```python
from build123d import *

# Parameters (mm, degrees)
SKETCH2_W           = 30
SKETCH2_H           = 30
BOSS_EXTRUDE1_DEPTH = 6.35
FILLET1_R           = 10
SKETCH3_R           = 6.5
BOSS_EXTRUDE2_DEPTH = 50
SKETCH4_R           = 0.5
BOSS_EXTRUDE3_DEPTH = 20
FILLET2_R           = 0.5
CHAMFER1_SIZE       = 6.5


with BuildPart() as part:
    # Sketch2 → Boss-Extrude1 (new body)
    with BuildSketch(Plane(origin=(0, 0, 0), x_dir=(1, 0, 0), z_dir=(0, 1, 0))):
        Rectangle(SKETCH2_W, SKETCH2_H)
    extrude(amount=BOSS_EXTRUDE1_DEPTH)

    # Fillet1
    fillet1_edges = [part.edges().sort_by_distance(p)[0] for p in [
        (-15, 3.175, 15),
        (-15, 3.175, -15),
        (15, 3.175, -15),
        (15, 3.175, 15),
    ]]
    fillet(fillet1_edges, radius=FILLET1_R)

    # Sketch3 → Boss-Extrude2 (add)
    with BuildSketch(Plane(origin=(0, 6.35, 0), x_dir=(1, 0, 0), z_dir=(0, 1, 0))):
        with Locations(Location((0, 0, 0), (0, 0, 270))):
            Circle(SKETCH3_R)
    extrude(amount=BOSS_EXTRUDE2_DEPTH)

    # Sketch4 → Boss-Extrude3 (add)
    with BuildSketch(Plane(origin=(0, 56.35, 0), x_dir=(1, 0, 0), z_dir=(0, 1, 0))):
        with Locations(Location((0, 0, 0), (0, 0, 270))):
            Circle(SKETCH4_R)
    extrude(amount=BOSS_EXTRUDE3_DEPTH)

    # Fillet2
    fillet2_edges = [part.edges().sort_by_distance(p)[0] for p in [
        (0, 76.35, -0.5),
    ]]
    fillet(fillet2_edges, radius=FILLET2_R)

    # Chamfer1
    # the kernel refuses this chamfer: 6.5 mm, written as the material it adds along each edge
    with BuildSketch(Plane(origin=(0, 56.35, 0), x_dir=(0, 0, 1), z_dir=(-1, 0, 0))) as chamfer1_piece_1_section:
        Polygon((0.5, CHAMFER1_SIZE), (0.5 + CHAMFER1_SIZE, 0), (0.5, 0), align=None)
    chamfer1_piece_1 = revolve(axis=Axis((0, 56.35, 0), (0, 1, 0)), mode=Mode.PRIVATE)
    chamfer1_piece_1 = chamfer1_piece_1 & Plane(origin=(0, 59.89101351, 0), x_dir=(0, 0, 1), z_dir=(0, -1, 0)) * Cylinder(6.5, 28, mode=Mode.PRIVATE)
    add(chamfer1_piece_1)


solid = part.part
```
Can you work these out from the model? Positions are in its coordinate system, mm. A direction names the side the tool comes from. Coordinates: 2 decimals unless noted, no trailing zeros. Order: outer loops, then holes, each group sorted by start corner. A loop starts at its lowest first (then second) coordinate and runs counter-clockwise, first axis right, second up.
1. For faces 1 (the face through (11.99, 3.22, 12.15)), 2 (the face through (0, 6.35, -7)), which set-ups out of +Z, -Z, +X, -X, +Y, -Y let a thin tool reach every point of the face, with its end or its side?
2. I'm going to push flat-ended pins straight in: pin 1 (8 mm diameter, centred on y = 37, z = 1, fed in from -X); pin 2 (5 mm diameter, centred on x = -3.5, y = 37, fed in from +Z); pin 3 (9 mm diameter, centred on x = -4.5, z = -1.5, fed in from +Y); pin 4 (6 mm diameter, centred on y = 27.5, z = 11, fed in from +X). Where does each tip first touch, or does it pass through?
3. If we section it at B-B (z = -13): Please give me the cut outline in (x, y), then the cut area to 3 significant figures.
4. If we section it at A-A (y = 50): Please give me the cut outline in (x, z), then the cut area to 3 significant figures.
5. I need wall thicknesses on line 1 (Y direction, x = -10, z = 9); line 2 (Z direction, x = 3.5, y = 23.5); line 3 (X direction, y = 41.5, z = -1.5). Which ranges of each line are inside material? Lowest first, please.
Entries:
1. face 1: +Z, +X, +Y, -Y
1. face 2: +Y
2. pin 1: stops at x = -6.5
2. pin 2: stops at z = 6.42
2. pin 3: stops at y = 76.29
2. pin 4: passes through
3. outline: (-11, 0) - (11, 0) - (11, 6.35) - (-11, 6.35) - close
3. area: 140 mm2
4. outline: circle Ø13 at (0, 0)
4. area: 133 mm2
5. line 1: y = 0 to 6.35
5. line 2: z = -5.48 to 5.48
5. line 3: x = -6.32 to 6.32
